Design review of the part built by this model. Coordinates are the model's own, in mm. A direction names the side the tool comes from. Coordinates: 2 decimals unless noted, no trailing zeros. Write each loop counter-clockwise with the first axis right and the second up, starting at its lowest first coordinate (ties: lowest second). Pieces come first, ordered by that corner, then holes. Notation, with made-up numbers: (-22, 78.5) - (-14, 78.5) arc R32 ccw to (-14, 113.5) - close; hole circle Ø10 at (36, 60.25). An arc over 180 degrees is marked (long way). Answer as a JSON object with one key per item and string values.
```python
from build123d import *

# Parameters (mm, degrees)
SKETCH_1_W      = 40
SKETCH_1_H      = 40
EXTRUDE_1_DEPTH = 20
SKETCH_5_R      = 1.5
EXTRUDE_2_DEPTH = 2
FILLET_1_R      = 2


with BuildPart() as part:
    # Эскиз1 → Бобышка-Вытянуть1 (new body, symmetric)
    with BuildSketch(Plane(origin=(0, 0, 0), x_dir=(1, 0, 0), z_dir=(0, 1, 0))):
        Rectangle(SKETCH_1_W, SKETCH_1_H)
    extrude(amount=EXTRUDE_1_DEPTH, both=True)

    # Эскиз4 → Вырез-Повернуть1 (revolve, cut)
    with BuildSketch(Plane.XY):
        Polygon((-4.5, -20), (-4.5, -19), (-8.75, -14.75), (-8.75, 19), (-9.75, 20), (0, 20), (0, -20), align=None)
    cut_revolve_1 = revolve(axis=Axis((0, 20, 0), (0, -1, 0)), mode=Mode.SUBTRACT)

    # Эскиз5 → Бобышка-Вытянуть2 (add)
    with BuildSketch(Plane.XZ.offset(20)):
        with Locations(Location((-15, 12.5, 0), (0, 0, 270))):  # turned: the seam where the file's is
            Circle(SKETCH_5_R)
        with Locations(Location((-15, -12.5, 0), (0, 0, 270))):  # turned: the seam where the file's is
            Circle(SKETCH_5_R)
        with Locations(Location((15, -12.5, 0), (0, 0, 270))):  # turned: the seam where the file's is
            Circle(SKETCH_5_R)
        with Locations(Location((15, 12.5, 0), (0, 0, 270))):  # turned: the seam where the file's is
            Circle(SKETCH_5_R)
    extrude_2 = extrude(amount=EXTRUDE_2_DEPTH)

    # Зеркальное отражение1: Вырез-Повернуть1, Бобышка-Вытянуть2 across plane
    add(cut_revolve_1.mirror(Plane(origin=(0, 0, 0), x_dir=(0, 0, 1), z_dir=(0.707106781, 0.707106781, 0))), mode=Mode.SUBTRACT)
    add(extrude_2.mirror(Plane(origin=(0, 0, 0), x_dir=(0, 0, 1), z_dir=(0.707106781, 0.707106781, 0))))

    # Скругление1
    fillet_1_edges = [part.edges().sort_by_distance(p)[0] for p in [
        (-20, 20, 0),
        (0, 20, 20),
        (20, 20, 0),
        (-20, -20, 0),
        (0, -20, -20),
        (-20, 0, 20),
        (-20, 0, -20),
        (20, 0, -20),
        (0, 20, -20),
    ]]
    fillet(fillet_1_edges, radius=FILLET_1_R)

    # Зеркальное отражение2: Вырез-Повернуть1, Бобышка-Вытянуть2 across plane
    add(cut_revolve_1.mirror(Plane(origin=(0, 0, 0), x_dir=(0, -0.707106781, 0.707106781), z_dir=(0, 0.707106781, 0.707106781))), mode=Mode.SUBTRACT)
    add(extrude_2.mirror(Plane(origin=(0, 0, 0), x_dir=(0, -0.707106781, 0.707106781), z_dir=(0, 0.707106781, 0.707106781))))


solid = part.part
```
(1) To check wall thickness, follow line 1 (Y direction, x = -15, z = 0). State the ranges of the line that lie inside material, in increasing order. Write a range as from..to.
Solved:
{"line 1": "y = -20..-8.75, 8.75..20"}
(2) The part is to be moulded in two halves that separate along Y. For faces 5 (the face through (8.74, 14.11, -0.38)), 6 (the face through (0.25, 19.43, -19.4)), 7 (the face through (15, 11, 21)), say which applies: pulls with the +Y half, pulls with the -Y half, needs draft (parallel to the pull), parting line crosses it, or undercut.
Solved:
{"face 5": "needs draft", "face 6": "pulls with the +Y half", "face 7": "undercut"}
(3) Tool access review of faces 1 (the face through (-15, -21, 14)), 2 (the face through (20.986, 13.735, -13.306)), 3 (the face through (1.27, 19.4, 19.43)), 4 (the face through (-15, -14, 21)): name each direction out of +Z, -Z, +X, -X, +Y, -Y from which nothing blocks a thin tool from reaching the whole face with its end or side.
Solved:
{"face 1": "-Y", "face 2": "+X", "face 3": "+Z, +X, -X, +Y", "face 4": "+Z"}
(4) Take a section at C-C, the plane y = 12.5. Write out the cut boundary in (x, z).
Solved:
{"outline": "(-20, -18) arc R2 ccw to (-18, -20) - (18, -20) arc R2 ccw to (20, -18) - (20, 20) - (16.5, 20) - (16.5, 22) - (13.5, 22) - (13.5, 20) - (-13.5, 20) - (-13.5, 22) - (-16.5, 22) - (-16.5, 20) - (-18, 20) arc R2 ccw to (-20, 18) - close; hole circle Ø17.5 at (0, 0)"}
(5) Take a section at D-D, the plane z = -12.5. Write out the cut boundary in (x, y).
Solved:
{"outline": "(-20, -18) arc R2 ccw to (-18, -20) - (-16.5, -20) - (-16.5, -22) - (-13.5, -22) - (-13.5, -20) - (13.5, -20) - (13.5, -22) - (16.5, -22) - (16.5, -20) - (20, -20) - (20, -16.5) - (22, -16.5) - (22, -13.5) - (20, -13.5) - (20, 13.5) - (22, 13.5) - (22, 16.5) - (20, 16.5) - (20, 18) arc R2 ccw to (18, 20) - (-18, 20) arc R2 ccw to (-20, 18) - close; hole circle Ø17.5 at (0, 0)"}
(6) For pin 1 (10.5 mm diameter, centred on x = 0, z = 0, fed in from -Y); pin 2 (5.5 mm diameter, centred on x = 0, z = 0, fed in from -Y); pin 3 (10.5 mm diameter, centred on y = 0, z = 0, fed in from -X); pin 4 (12 mm diameter, centred on y = -11.5, z = 4.5, fed in from +X), all flat-tipped, find the tip position at first contact; note any pin that passes through.
Solved:
{"pin 1": "stops at y = -20", "pin 2": "passes through", "pin 3": "stops at x = 18.25", "pin 4": "stops at x = 20"}
(7) Take a section at A-A, the plane y = 0. Give the number of separate pieces and of enclosed holes in the cut face, and give its area (3 significant figures).
Solved:
{"separate pieces": "4", "enclosed holes": "0", "area": "555 mm^2"}
